Source: CAD feature listing. Evaluate the final solid. Frame: model axes, mm. A direction names the side the tool comes from. Coordinates: 2 decimals unless noted, no trailing zeros. Loops run counter-clockwise (first coordinate to the right, second up) from the corner with the lowest first, then second, coordinate; pieces in that order, holes last. Notation, with made-up numbers: (75, -24.75) - (111, -24.75) arc R25 ccw to (111, 1.25) - close; hole circle Ø8 at (71, 79.5). An arc over 180 degrees is marked (long way). Use CSV: the item, a comma, the result in double quotes. Start each with the question number.
Autodesk Inventor part; units mm, degrees
ref_plane "YZ Plane" through (0, 0, 0) normal (1, 0, 0) x (0, 1, 0)
ref_plane "XZ Plane" through (0, 0, 0) normal (0, 1, 0) x (-1, 0, 0)
ref_plane "XY Plane" through (0, 0, 0) normal (0, 0, 1) x (1, 0, 0)
sketch "Sketch1" plane through (0, 0, 0) normal (0, 1, 0) x (-1, 0, 0)
  circle A0 centre (0, 0) radius 4.95
  dimension "d0" = 9.9
extrude "Extrusion1" add sketch "Sketch1" along normal mid plane 20
sketch "Sketch2" plane through (0, 0, 0) normal (0, 1, 0) x (-1, 0, 0)
  circle A0 centre (0, 0) radius 7
  dimension "d3" = 14
extrude "Extrusion2" add sketch "Sketch2" along normal mid plane 2
sketch "Sketch3" plane through (0, 10, 0) normal (0, 1, 0) x (1, 0, 0)
  line L0 (-12, 0) -> (13, 0)
  line L1 (13, 0) -> (13, 11)
  line L2 (13, 11) -> (-12, 11)
  line L3 (-12, 11) -> (-12, 0)
  point P0 (0, 0)
extrude "Extrusion3" cut sketch "Sketch3" against normal blind 28
properties part number "wall_pin"
(1) Section B-B on z = 4.5. Output: boundary loops of the cut face in (x, y), plus the area to 3 significant figures.
(2) Reachability of faces 1 (the flat face through (0, 10, 2)), 2 (the flat face through (0.1, 1, 5.1)), 3 (the flat face through (0.1, -1, 5.1)) from +Z, -Z, +X, -X, +Y, -Y: full face, straight path, thin tool, end or side. Return the list, or none.
(3) Pin query (flat end, axial travel): pin 1 Ø4 at (x, y) = (3, 5) entering from +Z; pin 2 Ø4 at (y, z) = (6.5, 2) entering from +X. Return the tip coordinate at first contact, or that it passes through.
(4) Ray query, line 1 (Y direction, x = 1.5, z = 5.5); line 2 (X direction, y = -4, z = 3.25); line 3 (Z direction, x = -2.25, y = 0.25). Return the intervals inside material, ascending. Write a range as [from, to].
(5) Section A-A on x = 0. Output: boundary loops of the cut face in (y, z).
(6) Section C-C on y = -6. Output: boundary loops of the cut face in (x, z), plus the area to 3 significant figures.
(7) Section D-D on x = -3.75. Output: boundary loops of the cut face in (y, z).
Solution:
1,outline,"(-5.36, -1) - (-2.06, -1) - (-2.06, -10) - (2.06, -10) - (2.06, -1) - (5.36, -1) - (5.36, 1) - (2.06, 1) - (2.06, 10) - (-2.06, 10) - (-2.06, 1) - (-5.36, 1) - close"
1,area,"95.7 mm²"
2,face 1,"+Z, -Z, +X, -X, +Y"
2,face 2,"+Z, +Y"
2,face 3,"+Z, -Y"
3,pin 1,"stops at z = 4.85"
3,pin 2,"stops at x = 4.95"
4,line 1,"y = [-1, 1]"
4,line 2,"x = [-3.73, 3.73]"
4,line 3,"z = [0, 6.63]"
5,outline,"(-10, 0) - (10, 0) - (10, 4.95) - (1, 4.95) - (1, 7) - (-1, 7) - (-1, 4.95) - (-10, 4.95) - close"
6,outline,"(-4.95, 0) - (4.95, 0) arc R4.95 ccw to start"
6,area,"38.5 mm²"
7,outline,"(-10, 0) - (10, 0) - (10, 3.23) - (1, 3.23) - (1, 5.91) - (-1, 5.91) - (-1, 3.23) - (-10, 3.23) - close"
